The figure shows three views and two pictorial views of one solid part (mm, origin at its lowest corner). Answer the questions. A direction names the side the tool comes from. Coordinates: 2 decimals unless noted, no trailing zeros. Order: outer loops, then holes, each group sorted by start corner. A loop starts at its lowest first (then second) coordinate and runs counter-clockwise, first axis right, second up. Notation, with made-up numbers: (83, -12) -> (95, -12) arc R15 cw to (95, 2) -> close; hole circle Ø10 at (-7.5, -15). An arc over 180 degrees is marked (long way). Write item = value, one per line. Start each with the question number.
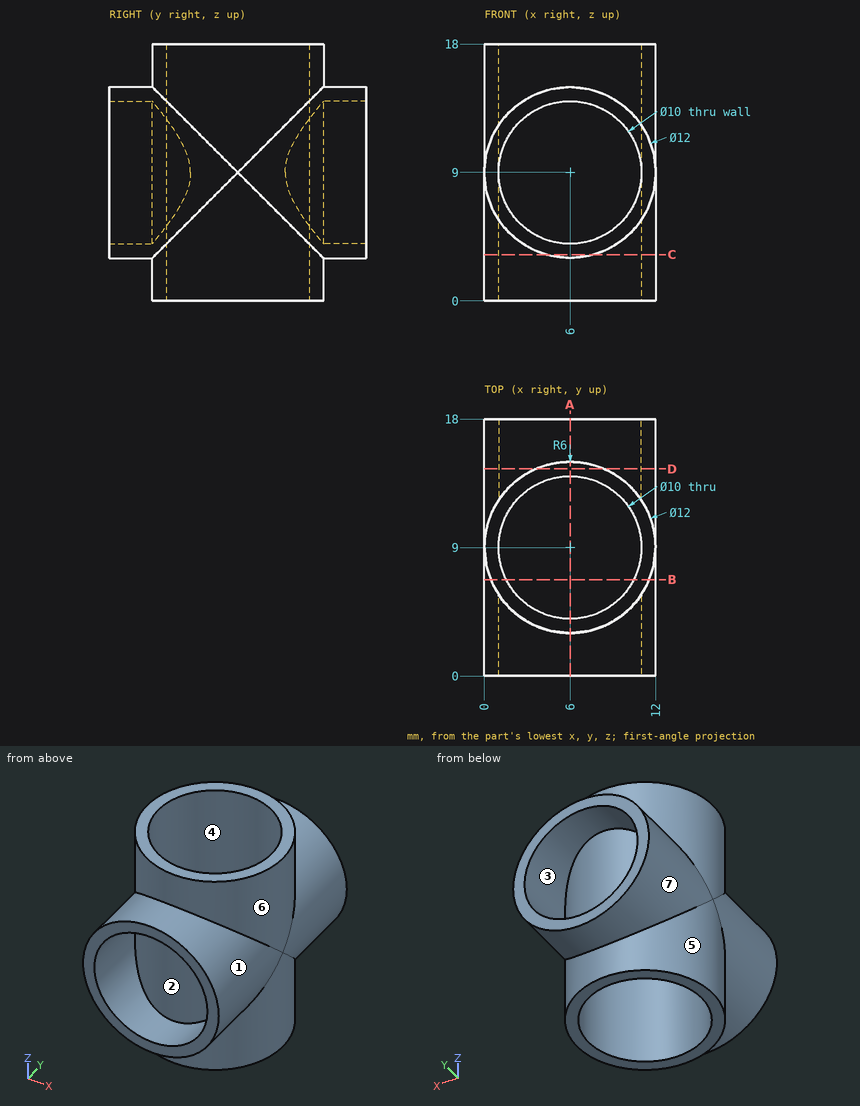
Item 1: Section B-B, the plane y = 6.75 is taken. Give the vertices of the cut face in (x, z), then the cut area to 3 significant figures.
Item 2: Which of the six approach directions +Z, -Z, +X, -X, +Y, -Y give full straight-line access (tool end or side, diameter ignored) to the marked faces 5, 6 and 7?
Item 3: Section A-A, the plane x = 6 is taken. Give the vertices of the cut face in (y, z), then the cut area to 3 significant figures.
Item 4: For a pull along Z with two mould halves and no side action, classify the marked faces 1, 2, 3 and 4 as pulls with the +Z half, pulls with the -Z half, needs draft (parallel to the pull), parting line crosses it, or undercut.
Item 5: Consider probe 1 along Y at (x, z) = (6, 13.25); probe 2 along X at (y, z) = (14.5, 9). Determine where each line is inside the solid, lowest interval first.
Item 6: Section D-D, the plane y = 14.5 is taken. Give the vertices of the cut face in (x, z).
Item 7: Each of these flat-tipped pins is pushed along its axis until it touches: pin 1 (4 mm diameter, centred on y = 7, z = 10.5, fed in from -X); pin 2 (1.5 mm diameter, centred on y = 4, z = 8, fed in from +X); pin 3 (1.5 mm diameter, centred on x = 3.5, z = 6, fed in from -Y); pin 4 (1.5 mm diameter, centred on x = 8, z = 12.5, fed in from -Y). Where does it stop, or does it pass through?
Item 8: Section C-C, the plane z = 3.25 is taken. Give the vertices of the cut face in (x, y), then the cut area to 3 significant figures.
A:
q1.outline = (0.44, 0) -> (1.53, 0) -> (1.53, 18) -> (0.44, 18) -> (0.44, 11.25) arc R6 ccw to (0.44, 6.75) -> close; (10.47, 0) -> (11.56, 0) -> (11.56, 6.75) arc R6 ccw to (11.56, 11.25) -> (11.56, 18) -> (10.47, 18) -> close
q1.area = 42.1 mm^2
q2.face_5 = -Z
q2.face_6 = +Z
q2.face_7 = +Y
q3.outline = (0, 3) -> (3, 3) -> (3, 0) -> (4, 0) -> (4, 18) -> (3, 18) -> (3, 15) -> (0, 15) -> (0, 14) -> (3, 14) -> (3, 4) -> (0, 4) -> close; (14, 0) -> (15, 0) -> (15, 3) -> (18, 3) -> (18, 4) -> (15, 4) -> (15, 14) -> (18, 14) -> (18, 15) -> (15, 15) -> (15, 18) -> (14, 18) -> close
q3.area = 48.0 mm^2
q4.face_1 = parting line crosses it
q4.face_2 = undercut
q4.face_3 = undercut
q4.face_4 = needs draft
q5.probe_1 = 3 to 4, 14 to 15
q5.probe_2 = 0 to 1, 3.6 to 8.4, 11 to 12
q6.outline = (3.6, 0) -> (8.4, 0) -> (8.4, 3.5) arc R6 ccw to (8.4, 14.5) -> (8.4, 18) -> (3.6, 18) -> (3.6, 14.5) arc R6 ccw to (3.6, 3.5) -> close; hole (3.6, 4.61) -> (3.6, 13.39) arc R5 ccw to start; hole (8.4, 4.61) arc R5 ccw to (8.4, 13.39) -> close
q7.pin_1 = 0
q7.pin_2 = 11.99
q7.pin_3 = 3.26
q7.pin_4 = 3.13
q8.outline = (4.29, 0) -> (7.71, 0) -> (7.71, 3.25) arc R6 ccw to (7.71, 14.75) -> (7.71, 18) -> (4.29, 18) -> (4.29, 14.75) arc R6 ccw to (4.29, 3.25) -> close; hole circle Ø10 at (6, 9)
q8.area = 55.7 mm^2
